Can you work these out from the drawing? Everything is in mm from the part's minimum corner. A direction names the side the tool comes from. Round coordinates to 2 decimals unless told otherwise and drop trailing zeros. Write each loop counter-clockwise with the first axis right and the second up, starting at its lowest first coordinate (ties: lowest second). Pieces come first, ordered by that corner, then holes. Notation, with made-up numbers: (64, 60.5) -> (89, 60.5) arc R21 cw to (89, 68.5) -> close; hole circle Ø9 at (61, -7.5). An arc over 180 degrees is marked (long way). Answer as CSV lines item,"result". Start each with the question number.
Q1. For the marked faces 1, 2, 3 and 4, which set-ups out of +Z, -Z, +X, -X, +Y, -Y let a thin tool reach every point of the face, with its end or its side?
Q2. Imagine slicing it at C-C on z = 28. Please give me the cut outline in (x, y).
Q3. Imagine slicing it at A-A on y = 40.64. Please give me the cut outline in (x, z), and give its area (3 significant figures).
Q4. Imagine slicing it at D-D on y = 58. Please give me the cut outline in (x, z).
Q5. Imagine slicing it at B-B on x = 97.79. Please give me the cut outline in (y, z), and give its area (3 significant figures).
Q6. Will these pins go through, and if not, where does the flat tip stop? pin 1 Ø10 at (x, y) = (139, 50) entering from +Z; pin 2 Ø7 at (y, z) = (47.5, 41) entering from +X; pin 3 Ø2 at (x, y) = (44, 17) entering from +Z.
Q7. If we mould it in two halves opening along X, with no side actions, what happens to the marked faces 5, 6 and 7? For each: pulls with the +X half, pulls with the -X half, needs draft (parallel to the pull), parting line crosses it, or undercut.
Q8. If I drill on line 1 (X direction, y = 40, z = 19); line 2 (Y direction, x = 97, z = 27); line 3 (Y direction, x = 45.72, z = 22.5), over which ranges is the centre line in solid material (lowest first)? Write a range as [from, to].
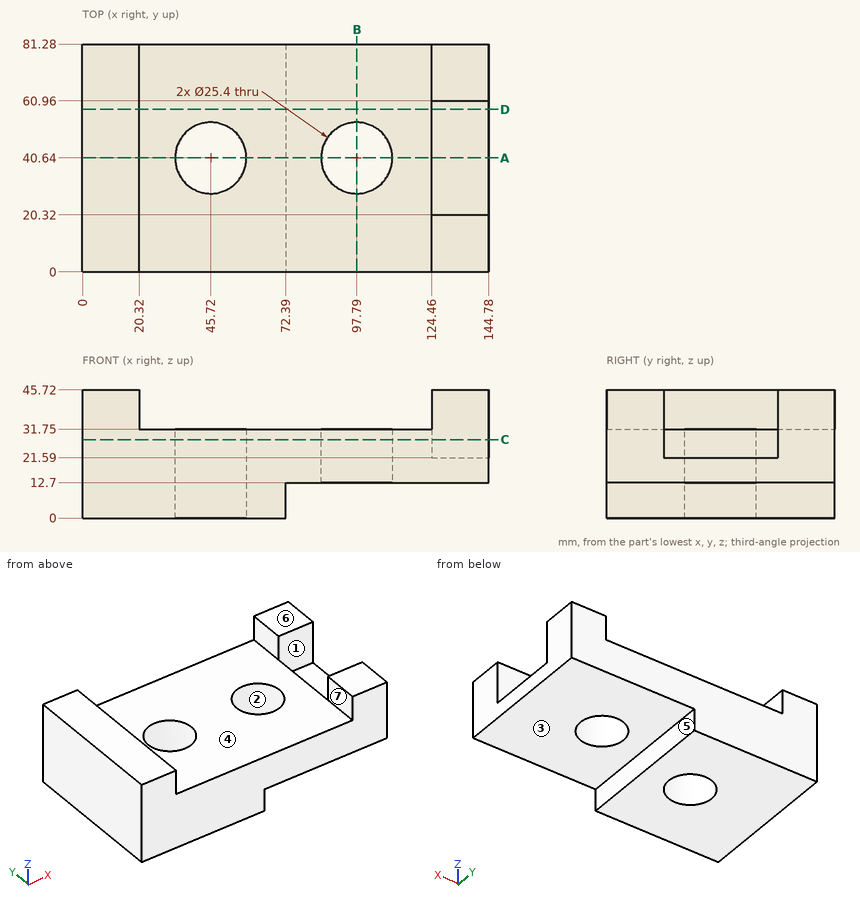
Checks:
1,face 1,"+Z, +X"
1,face 2,"+Z, -Z"
1,face 3,"-Z, +X, +Y, -Y"
1,face 4,"+Z, +Y, -Y"
2,outline,"(0, 0) -> (144.78, 0) -> (144.78, 20.32) -> (124.46, 20.32) -> (124.46, 60.96) -> (144.78, 60.96) -> (144.78, 81.28) -> (0, 81.28) -> close; hole circle Ø25.4 at (45.72, 40.64); hole circle Ø25.4 at (97.79, 40.64)"
3,outline,"(0, 0) -> (33.02, 0) -> (33.02, 31.75) -> (20.32, 31.75) -> (20.32, 45.72) -> (0, 45.72) -> close; (58.42, 0) -> (72.39, 0) -> (72.39, 12.7) -> (85.09, 12.7) -> (85.09, 31.75) -> (58.42, 31.75) -> close; (110.49, 12.7) -> (144.78, 12.7) -> (144.78, 21.59) -> (124.46, 21.59) -> (124.46, 31.75) -> (110.49, 31.75) -> close"
3,area,"2,460 mm^2"
4,outline,"(0, 0) -> (72.39, 0) -> (72.39, 12.7) -> (144.78, 12.7) -> (144.78, 21.59) -> (124.46, 21.59) -> (124.46, 31.75) -> (20.32, 31.75) -> (20.32, 45.72) -> (0, 45.72) -> close"
5,outline,"(0, 12.7) -> (27.94, 12.7) -> (27.94, 31.75) -> (0, 31.75) -> close; (53.34, 12.7) -> (81.28, 12.7) -> (81.28, 31.75) -> (53.34, 31.75) -> close"
5,area,"1,060 mm^2"
6,pin 1,"z = 21.59"
6,pin 2,"x = 20.32"
6,pin 3,"z = 31.75"
7,face 5,"pulls with the +X half"
7,face 6,"needs draft"
7,face 7,"undercut"
8,line 1,"[0, 33.04], [58.4, 85.11], [110.47, 144.78]"
8,line 2,"[0, 27.96], [53.32, 81.28]"
8,line 3,"[0, 27.94], [53.34, 81.28]"
